Build history of the part. All positions in model axes, mm. A direction names the side the tool comes from. Round coordinates to 2 decimals unless told otherwise and drop trailing zeros. Loops run counter-clockwise (first coordinate to the right, second up) from the corner with the lowest first, then second, coordinate; pieces in that order, holes last. Notation, with made-up numbers: M 63.5,11 L 76.5,11 A18 ccw 76.5,25 Z; hole C 73.5,-21 d1. An arc over 180 degrees is marked long. Use one line per item in the form item = value. Start each with the question number.
Autodesk Inventor part; units mm, degrees
ref_plane "YZ Plane" through (0, 0, 0) normal (1, 0, 0) x (0, 1, 0)
ref_plane "XZ Plane" through (0, 0, 0) normal (0, 1, 0) x (-1, 0, 0)
ref_plane "XY Plane" through (0, 0, 0) normal (0, 0, 1) x (1, 0, 0)
sketch "Esboço1" plane through (0, 0, 0) normal (0, 0, 1) x (1, 0, 0)
  line L0 (-22.5, 16.605) -> (22.5, 16.605) construction
  line L1 (22.5, 16.605) -> (22.5, -16.395) construction
  line L2 (22.5, -16.395) -> (-22.5, -16.395) construction
  line L3 (-22.5, -16.395) -> (-22.5, 16.605) construction
  line L4 (-14, 20.4248) -> (-14, -25.3484) construction
  line L5 (14, 20.4248) -> (14, -25.3484) construction
  line L6 (0, 20.9223) -> (0, -24.8509) construction
  line L7 (-26.3196, -3.395) -> (26.3196, -3.395) construction
  line L8 (-26.3196, 7.605) -> (26.3196, 7.605) construction
  line L9 (-21, 20.7786) -> (-21, -24.9946) construction
  line L10 (21, 20.4248) -> (21, -25.3484) construction
  line L11 (0, -3.395) -> (-21.4941, -29.0107) construction
  line L12 (0, -3.395) -> (21.8166, -29.395) construction
  line L13 (-10, 20.4248) -> (-10, -25.3484) construction
  line L14 (-5, 20.4248) -> (-5, -25.3484) construction
  line L15 (5, 20.9223) -> (5, -24.8509) construction
  line L16 (10, 20.9223) -> (10, -24.8509) construction
  line L17 (-26.3196, 5.605) -> (26.3196, 5.605) construction
  line L18 (-22.5, 16.605) -> (-22.5, 7.605)
  line L19 (-22.5, 7.605) -> (-21, 5.605)
  line L20 (-21, 5.605) -> (-21, -16.395)
  line L21 (-21, -16.395) -> (-10.9083, -16.395)
  line L22 (-10.9083, -16.395) -> (-8.999, -14.1196)
  line L23 (8.999, -14.1196) -> (10.9083, -16.395)
  line L24 (10.9083, -16.395) -> (21, -16.395)
  line L25 (22.5, 7.605) -> (22.5, 16.605)
  line L26 (26.3196, 14.605) -> (-26.3196, 14.605) construction
  line L27 (-22.5, 16.605) -> (-10, 16.605)
  line L28 (-5, 16.605) -> (5, 16.605)
  line L29 (22.5, 16.605) -> (10, 16.605)
  arc A0 (8.999, -14.1196) -> (-8.999, -14.1196) centre (0, -3.395) ccw
  line L30 (-10, 16.605) -> (-7.6714, 16.605) construction
  line L31 (-10, 16.605) -> (-9.0674, 14.605)
  line L32 (-10, 16.605) -> (-7.7932, 16.605) construction
  line L33 (-5, 16.605) -> (-5.9326, 14.605)
  line L34 (-5, 16.605) -> (-2.7932, 16.605) construction
  line L35 (-5.9326, 14.605) -> (-9.0674, 14.605)
  line L36 (5, 16.605) -> (5.9326, 14.605)
  line L37 (10, 16.605) -> (9.0674, 14.605)
  line L38 (5.9326, 14.605) -> (9.0674, 14.605)
  line L39 (21, -16.395) -> (21, 5.605)
  line L40 (22.5, 7.605) -> (21, 5.605)
  point P0 (0, 0)
  point P1 (0, 16.605)
  point P2 (0, 7.605)
  dimension "largura" = 45
  dimension "altura" = 33
  dimension "d2" = 14
  dimension "d3" = 14
  dimension "d4" = 20
  dimension "d5" = 9
  dimension "d7" = 1.5
  dimension "d8" = 1.5
  dimension "d9" = 40
  dimension "d10" = 40
  dimension "d11" = 5
  dimension "d12" = 5
  dimension "d13" = 10
  dimension "d14" = 10
  dimension "d15" = 2
  dimension "d16" = 2
  dimension "d18" = 14
  dimension "d21" = 115
  dimension "d22" = 115
  dimension "d23" = 115
  dimension "d24" = 115
extrude "Extrusão1" add sketch "Esboço1" along normal blind 45
chamfer "Chanfro1" distance 1.5 angle 45 4 edges at (22.5, 16.605, 22.5) (-22.5, 16.605, 22.5) (21, -16.395, 22.5) (-21, -16.395, 22.5)
sketch "Esboço2" plane through (-10, 16.605, 45) normal (0, 1, 0) x (1, 0, 0)
  line L0 (-12.5, 45) -> (-12.5, 0) construction
  line L1 (-12.5, 22.5) -> (32.5, 22.5) construction
  line L2 (32.5, 45) -> (32.5, 0) construction
  line L3 (10, 45) -> (10, 0) construction
  circle A0 centre (-6, 7.5) radius 1 construction
  circle A1 centre (26, 7.5) radius 1 construction
  circle A2 centre (-6, 37.5) radius 1 construction
  circle A3 centre (26, 37.5) radius 1 construction
  dimension "d31" = 2
  dimension "d32" = 2
  dimension "d33" = 2
  dimension "d34" = 2
  dimension "d35" = 16
  dimension "d36" = 16
  dimension "d37" = 16
  dimension "d38" = 16
  dimension "d39" = 15
  dimension "d40" = 15
  dimension "d41" = 15
  dimension "d42" = 15
hole "Furo1" at (-16, 16.605, 37.5) at (-16, 16.605, 7.5) at (16, 16.605, 7.5) at (16, 16.605, 37.5) direction (0, -1, 0) diameter 4.134 depth 8 tip angle 118
equation "\"d3\" = d2"
equation "\"d8\" = d7"
equation "\"d10\" = d9"
equation "\"d12\" = d11"
equation "\"d14\" = d13"
equation "\"d32\" = d31"
equation "\"d33\" = d31"
equation "\"d34\" = d31"
equation "\"d40\" = d39"
equation "\"d41\" = d39"
equation "\"d42\" = d39"
properties part number "PilowBlockAbertoSBR16"
Q1. Saw through at D-D (y = -2). Give the cut face in (x, z), and give its area (3 significant figures).
Q2. Saw through at A-A (z = 21). Give the cut face in (x, y) (3 decimals), and give its area (3 significant figures).
Q3. Pull direction X, two halves, no side cores. Call faces 1 (the face through (0, 11, 45)), 2 (the face through (5.46, 15.62, 22.18)), 3 (the face through (-22.5, 11, 22)): pulls with the +X half, pulls with the -X half, needs draft (parallel to the pull), parting line crosses it, or undercut.
Q4. Tool access for faces 4 (the face through (-7, 14.605, 22)), 5 (the face through (-9.967, -15.273, 22.185)), 6 (the face through (13.95, 12.55, 7.23)): list every direction of +Z, -Z, +X, -X, +Y, -Y with a clear straight run to the whole face (end or side of a thin tool).
Q5. Saw through at C-C (x = 0). Give the cut face in (y, z) (3 decimals), and give its area (3 significant figures).
Q6. Drop flat-ended pins along their axis: P1, Ø1.6, axis at x = 7, z = 16, coming from the +Y side (3 decimals); P2, Ø3.5, axis at x = -7, z = 32.5, coming from the +Y side; P3, Ø10, axis at y = -3.5, z = 20, coming from the -X side. Give the stop position or say it passes through.
Q7. Saw through at B-B (y = 5). Give the cut face in (x, z).
Q8. Wall check: probe 1 along Z at (x, y) = (-16, 12); probe 2 along X at (y, z) = (13.5, 37.5); probe 3 along X at (y, z) = (-2, 4). Give the ranges that are in metal, low to high.
Filled in:
q1.outline = M -21,0 L -13.93,0 L -13.93,45 L -21,45 Z; M 13.93,0 L 21,0 L 21,45 L 13.93,45 Z
q1.area = 636 mm²
q2.outline = M -22.5,7.605 L -21,5.605 L -21,-14.895 L -19.5,-16.395 L -10.908,-16.395 L -8.999,-14.12 A14 cw long 8.999,-14.12 L 10.908,-16.395 L 19.5,-16.395 L 21,-14.895 L 21,5.605 L 22.5,7.605 L 22.5,15.105 L 21,16.605 L 10,16.605 L 9.067,14.605 L 5.933,14.605 L 5,16.605 L -5,16.605 L -5.933,14.605 L -9.067,14.605 L -10,16.605 L -21,16.605 L -22.5,15.105 Z
q2.area = 775 mm²
q3.face_1 = needs draft
q3.face_2 = undercut
q3.face_3 = pulls with the -X half
q4.face_4 = +Z, -Z, +Y
q4.face_5 = +Z, -Z, -Y
q4.face_6 = +Y
q5.outline = M 10.605,0 L 16.605,0 L 16.605,45 L 10.605,45 Z
q5.area = 270 mm²
q6.P1 = 14.605
q6.P2 = 16.07
q6.P3 = -21
q7.outline = M -21,0 L -11.2,0 L -11.2,45 L -21,45 Z; M 11.2,0 L 21,0 L 21,45 L 11.2,45 Z
q8.probe_1 = 0 to 5.43, 9.57 to 35.43, 39.57 to 45
q8.probe_2 = -22.5 to -18.07, -13.93 to 13.93, 18.07 to 22.5
q8.probe_3 = -21 to -13.93, 13.93 to 21
